Can you work these out from the model? Positions are in its coordinate system, mm. Face numbers are marked on the shaded views. A direction names the side the tool comes from. Coordinates: 2 decimals unless noted, no trailing zeros. Order: outer loops, then holes, each group sorted by start corner. A loop starts at its lowest first (then second) coordinate and runs counter-clockwise, first axis right, second up.
```python
from build123d import *

# Parameters (mm, degrees)
SKETCH_1_R          = 35
EXTRUDE_1_DEPTH     = 5
SKETCH_2_R          = 23.5
EXTRUDE_2_DEPTH     = 10
SKETCH_3_R          = 20
CUT_EXTRUDE_1_DEPTH = 14
SKETCH_4_R          = 3
CUT_EXTRUDE_2_DEPTH = 14
CHAMFER_1_SIZE      = 0.5


with BuildPart() as part:
    # 草图1 → 凸台-拉伸1 (new body)
    with BuildSketch(Plane(origin=(0, 0, 0), x_dir=(1, 0, 0), z_dir=(0, 1, 0))):
        with Locations(Location((0, 0, 0), (0, 0, 270))):
            Circle(SKETCH_1_R)
    extrude(amount=EXTRUDE_1_DEPTH)

    # 草图2 → 凸台-拉伸2 (add)
    with BuildSketch(Plane(origin=(0, 5, 0), x_dir=(1, 0, 0), z_dir=(0, 1, 0))):
        with Locations(Location((0, 0, 0), (0, 0, 270))):
            Circle(SKETCH_2_R)
    extrude(amount=EXTRUDE_2_DEPTH)

    # 草图3 → 切除-拉伸1 (cut)
    with BuildSketch(Plane.XZ):
        with Locations(Location((0, 0, 0), (0, 0, 270))):
            Circle(SKETCH_3_R)
    extrude(amount=-CUT_EXTRUDE_1_DEPTH, mode=Mode.SUBTRACT)

    # 草图4 → 切除-拉伸2 (cut)
    with BuildSketch(Plane(origin=(0, 5, 0), x_dir=(1, 0, 0), z_dir=(0, 1, 0))):
        with Locations(Location((0, 30, 0), (0, 0, 270))):
            Circle(SKETCH_4_R)
        with Locations(Location((25.980762114, 15, 0), (0, 0, 270))):
            Circle(SKETCH_4_R)
        with Locations(Location((25.980762114, -15, 0), (0, 0, 270))):
            Circle(SKETCH_4_R)
        with Locations(Location((0, -30, 0), (0, 0, 270))):
            Circle(SKETCH_4_R)
        with Locations(Location((-25.980762114, -15, 0), (0, 0, 270))):
            Circle(SKETCH_4_R)
        with Locations(Location((-25.980762114, 15, 0), (0, 0, 270))):
            Circle(SKETCH_4_R)
    extrude(amount=-CUT_EXTRUDE_2_DEPTH, mode=Mode.SUBTRACT)

    # Chamfer 1
    chamfer_1_edges = [part.edges().sort_by_distance(p)[0] for p in [
        (0, 0, 20),
        (0, 0, -35),
        (0, 5, -35),
        (0, 15, -23.5),
    ]]
    chamfer(chamfer_1_edges, length=CHAMFER_1_SIZE)


solid = part.part
```
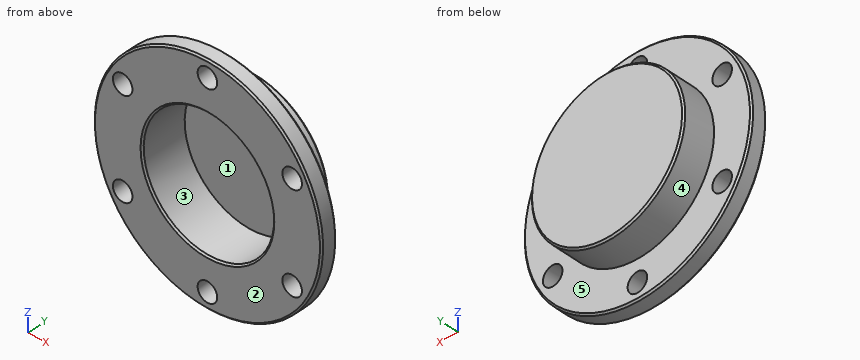
1. Please list where these lines run through material, in increasing order: probe 1 along X at (y, z) = (1.35, -15); probe 2 along X at (y, z) = (5.5, 0); probe 3 along Y at (x, z) = (-1.5, -3.5).
Completed:
probe 1: x = -31.62 to -28.98, -22.98 to -13.23, 13.23 to 22.98, 28.98 to 31.62
probe 2: x = -23.5 to -20, 20 to 23.5
probe 3: y = 14 to 15
2. Imagine slicing it at C-C on y = 3.5. Please give me the cut outline in (x, z), then the cut area to 3 significant figures.
Completed:
outline: circle Ø70 at (0, 0); hole circle Ø6 at (-25.98, -15); hole circle Ø6 at (-25.98, 15); hole circle Ø40 at (0, 0); hole circle Ø6 at (0, -30); hole circle Ø6 at (0, 30); hole circle Ø6 at (25.98, -15); hole circle Ø6 at (25.98, 15)
area: 2,420 mm2
3. Imagine slicing it at A-A on x = 0. Please give me the cut outline in (y, z).
Completed:
outline: (0, -34.5) - (0.5, -35) - (4.5, -35) - (5, -34.5) - (5, -33) - (0, -33) - close; (0, -27) - (5, -27) - (5, -23.5) - (14.5, -23.5) - (15, -23) - (15, 23) - (14.5, 23.5) - (5, 23.5) - (5, 27) - (0, 27) - (0, 20.5) - (0.5, 20) - (14, 20) - (14, -20) - (0.5, -20) - (0, -20.5) - close; (0, 33) - (5, 33) - (5, 34.5) - (4.5, 35) - (0.5, 35) - (0, 34.5) - close
4. On a 3-axis mill with a long thin cutter (end or side, diameter ignored), from which of +Z, -Z, +X, -X, +Y, -Y can I reach the whole of each face in a straight line? I mean the marked faces 1 and 2. Say none if no direction works.
Completed:
face 1: -Y
face 2: +Z, -Z, +X, -X, -Y
5. I'm going to push flat-ended pins straight in: pin 1 (6 mm diameter, centred on x = 1, y = 12, fed in from -Z); pin 2 (7 mm diameter, centred on x = 0, z = -30, fed in from +Y); pin 3 (4 mm diameter, centred on y = 2, z = -3, fed in from -X). Where does each tip first touch, or does it pass through?
Completed:
pin 1: stops at z = -23.5
pin 2: stops at y = 5
pin 3: stops at x = -34.99
6. Imagine slicing it at B-B on z = 0. Please give me the cut outline in (x, y), then the cut area to 3 significant figures.
Completed:
outline: (-35, 0.5) - (-34.5, 0) - (-20.5, 0) - (-20, 0.5) - (-20, 14) - (20, 14) - (20, 0.5) - (20.5, 0) - (34.5, 0) - (35, 0.5) - (35, 4.5) - (34.5, 5) - (23.5, 5) - (23.5, 14.5) - (23, 15) - (-23, 15) - (-23.5, 14.5) - (-23.5, 5) - (-34.5, 5) - (-35, 4.5) - close
area: 259 mm2
7. Thinking about a two-plate mould opening in X: for the marked faces 3, 4 and 5, which applies, pulls with the +X half, pulls with the -X half, needs draft (parallel to the pull), parting line crosses it, or undercut?
Completed:
face 3: undercut
face 4: parting line crosses it
face 5: needs draft
8. Imagine slicing it at D-D on y = 8.5. Please give me the cut outline in (x, z), then the cut area to 3 significant figures.
Completed:
outline: circle Ø47 at (0, 0); hole circle Ø40 at (0, 0)
area: 478 mm2
